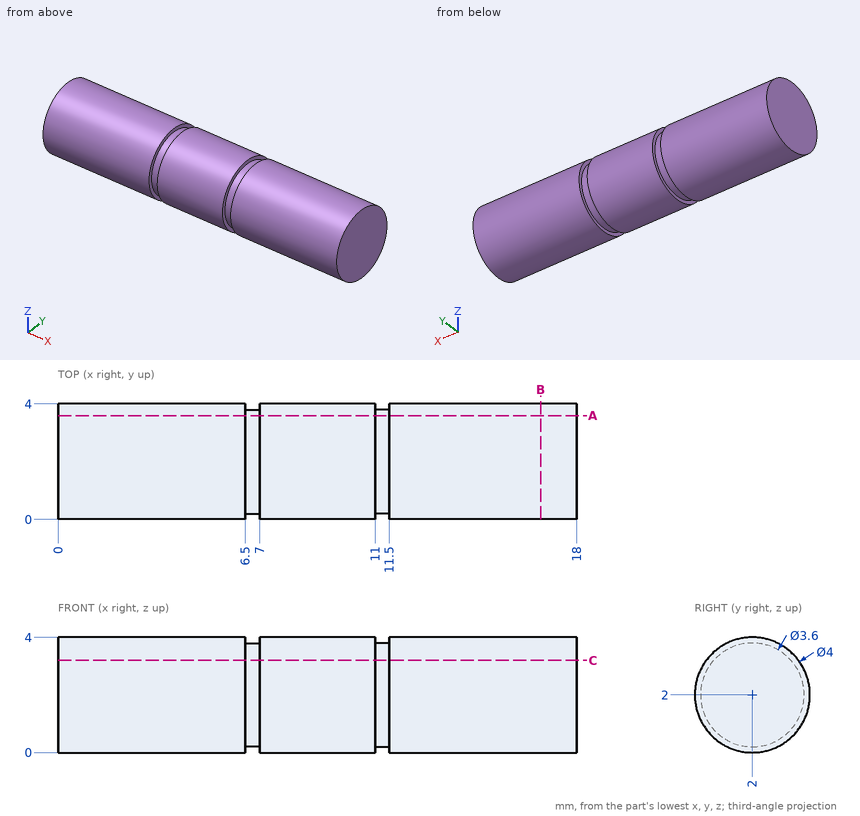
Design review of the part shown in the three views and the two pictorial views. Dimensions are in mm from the part's minimum x, y and z. Round coordinates to 2 decimals unless told otherwise and drop trailing zeros. Write each loop counter-clockwise with the first axis right and the second up, starting at its lowest first coordinate (ties: lowest second). Pieces come first, ordered by that corner, then holes. Notation, with made-up numbers: (-8, 12) - (8, 12) arc R7 ccw to (8, 20) - close; hole circle Ø1 at (47, 17). An arc over 180 degrees is marked (long way). Return JSON: item names as keys, results as strings. Group by question number.
Item 1: For probe 1 along X at (y, z) = (0.3, 1.25); probe 2 along Z at (x, y) = (16, 2.1), list the stretches that pass through material, from the lowest coordinate up. Write a range as [from, to].
Item 2: We need section C-C on z = 3.2. Write out the cut boundary in (x, y).
Item 3: Insertion check: P1, Ø2, axis at y = 1, z = 3, coming from the -X side; P2, Ø1.5, axis at x = 8, y = 3, coming from the -Z side. Each pin has a flat end and moves straight along its axis. Give the tip position at first contact, or say it passes through.
Item 4: We need section B-B on x = 16.75. Write out the cut boundary in (y, z), and give its area (3 significant figures).
Item 5: We need section A-A on y = 3.6. Write out the cut boundary in (x, z), and give its area (3 significant figures).
Model answer:
{
 "1": {"probe 1": "x = [0, 6.5], [7, 11], [11.5, 18]", "probe 2": "z = [0, 4]"},
 "2": {"outline": "(0, 0.4) - (6.5, 0.4) - (6.5, 0.66) - (7, 0.66) - (7, 0.4) - (11, 0.4) - (11, 0.66) - (11.5, 0.66) - (11.5, 0.4) - (18, 0.4) - (18, 3.6) - (11.5, 3.6) - (11.5, 3.34) - (11, 3.34) - (11, 3.6) - (7, 3.6) - (7, 3.34) - (6.5, 3.34) - (6.5, 3.6) - (0, 3.6) - close"},
 "3": {"P1": "stops at x = 0", "P2": "stops at z = 0.02"},
 "4": {"outline": "circle Ø4 at (2, 2)", "area": "12.6 mm²"},
 "5": {"outline": "(0, 0.8) - (6.5, 0.8) - (6.5, 1.18) - (7, 1.18) - (7, 0.8) - (11, 0.8) - (11, 1.18) - (11.5, 1.18) - (11.5, 0.8) - (18, 0.8) - (18, 3.2) - (11.5, 3.2) - (11.5, 2.82) - (11, 2.82) - (11, 3.2) - (7, 3.2) - (7, 2.82) - (6.5, 2.82) - (6.5, 3.2) - (0, 3.2) - close", "area": "42.4 mm²"}
}
